from build123d import *

# Parameters (mm, degrees)
F1_DEPTH       = 35
F3_D           = 5
F3_START       = 1.7550021
F3_CBORE_D     = 10
F3_CBORE_DEPTH = 8
F5_W           = 22.4
F5_H           = 2
F6_DEPTH       = 25
F7_R           = 6
F8_DEPTH       = 8


with BuildPart() as f1:
    # F0 (on Top) → F1 (new body, symmetric)
    with BuildSketch(Plane.XY):
        with BuildLine():
            ThreePointArc((-17.3192642082, 2.5086026559), (17.5, 0), (-17.3192642082, -2.5086026559))
            Line((-17.3192642082, -2.5086026559), (-28.1192642082, -2.5086026559))
            Line((-28.1192642082, -2.5086026559), (-28.1192642082, -10.9086026559))
            ThreePointArc((-28.1192642082, -10.9086026559), (-25.7761184577, -16.5654569054), (-20.1192642082, -18.9086026559))
            Line((-20.1192642082, -18.9086026559), (-7.9192642082, -18.9086026559))
            ThreePointArc((-7.9192642082, -18.9086026559), (20.5, 0), (-7.9192642082, 18.9086026559))
            Line((-7.9192642082, 18.9086026559), (-20.1192642082, 18.9086026559))
            ThreePointArc((-20.1192642082, 18.9086026559), (-25.7761184577, 16.5654569054), (-28.1192642082, 10.9086026559))
            Line((-28.1192642082, 10.9086026559), (-28.1192642082, 2.5086026559))
            Line((-28.1192642082, 2.5086026559), (-17.3192642082, 2.5086026559))
        make_face()
    extrude(amount=F1_DEPTH, both=True)

    # F3 (through all)
    # its depths count from where the whole tool has entered the part; down to there all is cleared
    with Locations(Plane(origin=(0, 18.9086026559, 0), x_dir=(-1, 0, 0), z_dir=(0, 1, 0)).offset(-F3_START)):
        with Locations((20.1192642082, 21.5039052665), (20.1192642082, 6.5039052665), (20.1192642082, -26.9960947335), (20.1192642082, -11.9960947335)):
            CounterBoreHole(F3_D / 2, F3_CBORE_D / 2, F3_CBORE_DEPTH)

    # F5 (on Front) → F6 (cut, symmetric)
    with BuildSketch(Plane.XZ):
        with Locations((-16.9192642082, -1)):
            Rectangle(F5_W, F5_H)
    extrude(amount=F6_DEPTH, both=True, mode=Mode.SUBTRACT)

    # F7 (on face) → F8 (cut)
    with BuildSketch(Plane.XY.offset(35)):
        with Locations((0, -25)):
            Circle(F7_R)
        with Locations((17.6776695297, -17.6776695297)):
            Circle(F7_R)
        with Locations((25, 0)):
            Circle(F7_R)
        with Locations((17.6776695297, 17.6776695297)):
            Circle(F7_R)
        with Locations((0, 25)):
            Circle(F7_R)
    extrude(amount=-F8_DEPTH, mode=Mode.SUBTRACT)


solid = f1.part
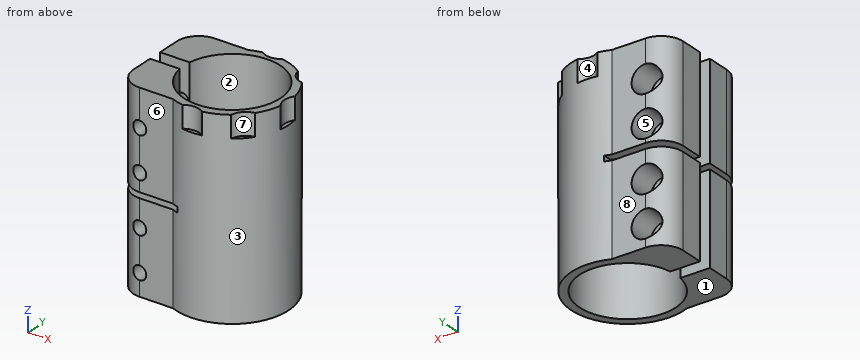
Design review of the part built by this model. Coordinates are the model's own, in mm. Face numbers are marked on the shaded views. A direction names the side the tool comes from. Round coordinates to 2 decimals unless told otherwise and drop trailing zeros. Loops run counter-clockwise (first coordinate to the right, second up) from the corner with the lowest first, then second, coordinate; pieces in that order, holes last. Notation, with made-up numbers: M 11.5,-6 L 60.5,-6 A9 ccw 60.5,6 Z; hole C 83,4 d1. An arc over 180 degrees is marked long. Answer as a JSON object with one key per item and string values.
Item 1: The part is to be moulded in two halves that separate along Y. For the marked faces 1, 2, 3 and 4, say which applies: pulls with the +Y half, pulls with the -Y half, needs draft (parallel to the pull), parting line crosses it, or undercut.
Answer sheet:
{"face 1": "needs draft", "face 2": "undercut", "face 3": "parting line crosses it", "face 4": "pulls with the +Y half"}
Item 2: We need section B-B on y = 15. Give the boundary of the cut face in (x, z).
Answer sheet:
{"outline": "M -26.99,-35 L -9.01,-35 L -9.01,-2 L -26.99,-2 Z; M -26.99,0 L -9.01,0 L -9.01,35 L -26.99,35 Z; M 9.01,-35 L 13.97,-35 L 13.97,27 L 12.31,27 L 12.31,35 L 9.01,35 Z; hole C -20.12,-27 d10; hole C -20.12,-12 d10; hole C -20.12,6.5 d10; hole C -20.12,21.5 d10"}
Item 3: We need section C-C on z = -21. Give the boundary of the cut face in (x, y), and give its area (3 significant figures).
Answer sheet:
{"outline": "M -28.12,-10.91 A8 ccw -20.12,-18.91 L -7.92,-18.91 A20.5 ccw long -7.92,18.91 L -20.12,18.91 A8 ccw -28.12,10.91 L -28.12,2.51 L -17.32,2.51 A17.5 cw long -17.32,-2.51 L -28.12,-2.51 Z", "area": "697 mm^2"}
Item 4: We need section D-D on y = 0. Give the boundary of the cut face in (x, z), and give its area (3 significant figures).
Answer sheet:
{"outline": "M 17.5,-35 L 20.5,-35 L 20.5,27 L 19,27 L 19,35 L 17.5,35 Z", "area": "198 mm^2"}
Item 5: Clearance check with flat-ended pins moving along their axes: P1, Ø1, axis at y = 9, z = -27.5, coming from the +X side; P2, Ø2, axis at x = 7, z = 13.5, coming from the +Y side; P3, Ø9, axis at x = -20.12, z = -27, coming from the -Y side. State where each tip first meets the part, or that it passes through.
Answer sheet:
{"P1": "stops at x = 18.65", "P2": "stops at y = 19.6", "P3": "stops at y = -18.91"}
Item 6: We need section A-A on x = 0. Give the boundary of the cut face in (y, z), and give its area (3 significant figures).
Answer sheet:
{"outline": "M -20.5,-35 L -17.5,-35 L -17.5,35 L -19,35 L -19,27 L -20.5,27 Z; M 17.5,-35 L 20.5,-35 L 20.5,27 L 19,27 L 19,35 L 17.5,35 Z", "area": "396 mm^2"}
Item 7: Wall thickness on L1, parallel to Z at x = -26, y = 5.5; L2, parallel to Y at x = -18, z = 28; L3, parallel to Z at x = -22, y = 3: over which ranges is each line inside the solid? List them lowest first. Write a range as from..to.
Answer sheet:
{"L1": "z = -35..-2, 0..35", "L2": "y = -18.91..-2.51, 2.51..18.91", "L3": "z = -35..-28.64, -25.35..-13.64, -10.35..-2, 0..4.86, 8.15..19.86, 23.15..35"}
Item 8: Machinability: for the marked faces 5, 6, 7 and 8, which of the approach directions +Z, -Z, +X, -X, +Y, -Y give a long, thin tool a straight path to every point of the face, cutting with its end or side? Answer none if there is none.
Answer sheet:
{"face 5": "+Y", "face 6": "+Z, -Z, -X, -Y", "face 7": "+Z, +X, -Y", "face 8": "+Z, -Z, -X, +Y"}
